Here's the drawing with two shaded views (mm, measured from the low corner). I have some questions. Coordinates: 2 decimals unless noted, no trailing zeros. Write each loop counter-clockwise with the first axis right and the second up, starting at its lowest first coordinate (ties: lowest second). Pieces come first, ordered by that corner, then holes.
Item 1: If we section it at C-C (x = 84.5): Please give me the cut outline in (y, z).
Item 2: If I drill on line 1 (Z direction, x = 109, y = 3.15); line 2 (Z direction, x = 81, y = 4.45); line 3 (X direction, y = 0.45, z = 26), over which ranges is the centre line in solid material (lowest first)?
Item 3: If we section it at B-B (z = 116): Please give me the cut outline in (x, y), then the cut area to 3 significant figures.
Item 4: If we section it at A-A (x = 50): Please give me the cut outline in (y, z).
Item 5: I'm going to push flat-ended pins straight in: pin 1 Ø3 at (y, z) = (2.5, 26.5) entering from -X; pin 2 Ø3 at (x, y) = (3, 4.5) entering from -Z; pin 3 Ø3 at (x, y) = (34, 3.5) entering from +Z; pin 4 Ø3 at (y, z) = (2.5, 170) entering from +X. Where does each tip first touch, or does it pass through?
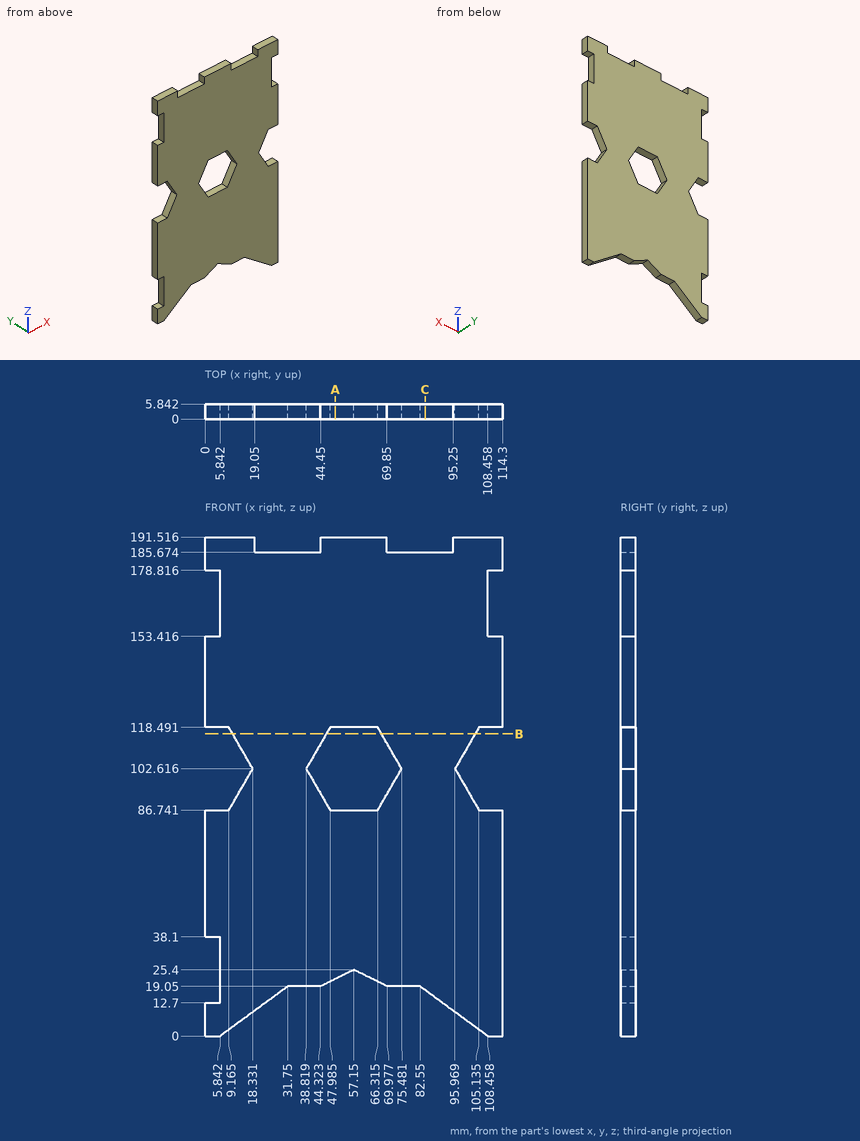
Answer list:
1. outline: (0, 17.62) - (5.84, 17.62) - (5.84, 185.67) - (0, 185.67) - close
2. line 1: z = 0 to 86.74, 118.49 to 153.42, 178.82 to 191.52
2. line 2: z = 19.05 to 185.67
2. line 3: x = 5.84 to 114.3
3. outline: (10.6, 0) - (46.55, 0) - (46.55, 5.84) - (10.6, 5.84) - close; (67.75, 0) - (103.7, 0) - (103.7, 5.84) - (67.75, 5.84) - close
3. area: 420 mm2
4. outline: (0, 21.86) - (5.84, 21.86) - (5.84, 86.74) - (0, 86.74) - close; (0, 118.49) - (5.84, 118.49) - (5.84, 191.52) - (0, 191.52) - close
5. pin 1: stops at x = 5.84
5. pin 2: stops at z = 0
5. pin 3: stops at z = 185.67
5. pin 4: stops at x = 108.46
